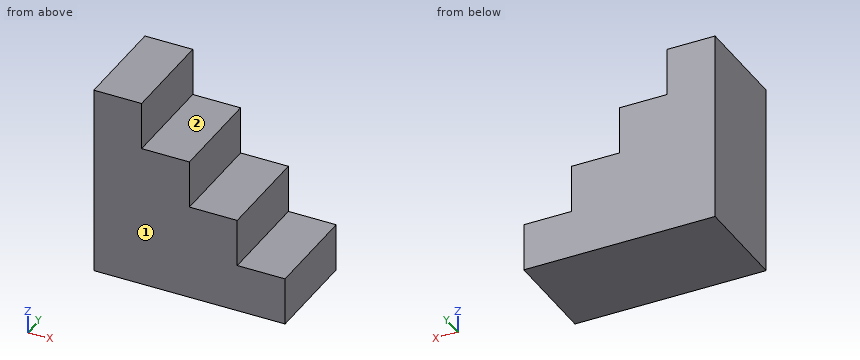
from build123d import *

# Parameters (mm, degrees)
F0_W     = 476.25
F0_H     = 914.4
F1_DEPTH = 228.6
F2_W     = 476.25
F2_H     = 685.8
F3_DEPTH = 228.6
F4_W     = 476.25
F4_H     = 457.2
F5_DEPTH = 228.6
F6_W     = 476.25
F6_H     = 228.6
F7_DEPTH = 228.6


with BuildPart() as f1:
    # F0 (on Right) → F1 (new body)
    with BuildSketch(Plane.YZ):
        with Locations((-18.221811, 93.697212)):
            Rectangle(F0_W, F0_H)
    extrude(amount=F1_DEPTH)

    # F2 (on face) → F3 (join)
    with BuildSketch(Plane.YZ.offset(228.6)):
        with Locations((-18.221811, -20.602788)):
            Rectangle(F2_W, F2_H)
    extrude(amount=F3_DEPTH)

    # F4 (on face) → F5 (join)
    with BuildSketch(Plane.YZ.offset(457.2)):
        with Locations((-18.221811, -134.902788)):
            Rectangle(F4_W, F4_H)
    extrude(amount=F5_DEPTH)

    # F6 (on face) → F7 (join)
    with BuildSketch(Plane.YZ.offset(685.8)):
        with Locations((-18.221811, -249.202788)):
            Rectangle(F6_W, F6_H)
    extrude(amount=F7_DEPTH)


solid = f1.part
Can you work these out from the model? Positions are in its coordinate system, mm. Face numbers are marked on the shaded views. A direction names the side the tool comes from. Coordinates: 2 decimals unless noted, no trailing zeros. Loops run counter-clockwise (first coordinate to the right, second up) from the corner with the lowest first, then second, coordinate; pieces in that order, holes last. Notation, with made-up numbers: M -33.5,-28.5 L -29.5,-28.5 A23 ccw -29.5,-6.5 Z; hole C 36,-21 d9. An arc over 180 degrees is marked long. Return JSON: item names as keys, results as strings. Group by question number.
Item 1: On a 3-axis mill with a long thin cutter (end or side, diameter ignored), from which of +Z, -Z, +X, -X, +Y, -Y can I reach the whole of each face in a straight line? I mean the marked faces 1 and 2. Say none if no direction works.
Item 2: Imagine slicing it at B-B (z = -103.5). Please give me the cut outline in (x, y).
Item 3: Imagine slicing it at A-A (y = 182). Please give me the cut outline in (x, z).
Item 4: Imagine slicing it at C-C (x = 533). Please give me the cut outline in (y, z), and give its area (3 significant figures).
Item 5: If I drill on L1, parallel to X at y = -26.5, z = 373; L2, parallel to X at y = -182, z = -40; L3, parallel to Z at x = 368.5, y = -65, over which ranges is the centre line in solid material (lowest first)? Write a range as from..to.
Item 6: I'm going to push flat-ended pins straight in: pin 1 Ø4 at (x, y) = (625.5, -79) entering from +Z; pin 2 Ø5 at (y, z) = (61.5, -208) entering from -X. Where does each tip first touch, or does it pass through?
Verdict:
{
 "1": {"face 1": "+Z, -Z, +X, -X, -Y", "face 2": "+Z, +X, +Y, -Y"},
 "2": {"outline": "M 0,-256.35 L 685.8,-256.35 L 685.8,219.9 L 0,219.9 Z"},
 "3": {"outline": "M 0,-363.5 L 914.4,-363.5 L 914.4,-134.9 L 685.8,-134.9 L 685.8,93.7 L 457.2,93.7 L 457.2,322.3 L 228.6,322.3 L 228.6,550.9 L 0,550.9 Z"},
 "4": {"outline": "M -256.35,-363.5 L 219.9,-363.5 L 219.9,93.7 L -256.35,93.7 Z", "area": "218,000 mm^2"},
 "5": {"L1": "x = 0..228.6", "L2": "x = 0..685.8", "L3": "z = -363.5..322.3"},
 "6": {"pin 1": "stops at z = 93.7", "pin 2": "stops at x = 0"}
}
